Build history of the part. All positions in model axes, mm. A direction names the side the tool comes from. Round coordinates to 2 decimals unless told otherwise and drop trailing zeros. Write each loop counter-clockwise with the first axis right and the second up, starting at its lowest first coordinate (ties: lowest second). Pieces come first, ordered by that corner, then holes.
1) Flat gauge pins, fed straight in: pin 1 (1 mm diameter, centred on y = -5, z = 2, fed in from +X); pin 2 (10 mm diameter, centred on x = -15, y = 15, fed in from -Z); pin 3 (3 mm diameter, centred on x = 0, y = 0, fed in from -Z). Where does each tip first touch, or does it go through?
2) Pull direction X, two halves, no side cores. Call faces 1 (the cylindrical face through (9.977, 15.656, 1.282)), 2 (the cylindrical face through (14.54, -18.62, 1.28)), 3 (the cylindrical face through (-23.598, 1.206, 1.282)): +X half, -X half, draft (parallel to the pull), parting line (faces both ways), or undercut.
3) Saw through at A-A (x = 0). Write the cut outline in (y, z), plus the area to 3 significant figures.
4) Which spindle directions (+Z, -Z, +X, -X, +Y, -Y) get a long thin tool onto all of the face, cutting with end or side? Do faces 4 (the cylindrical face through (-10.9, -20.965, 1.282)), 5 (the cylindrical face through (8.71, 22.02, 1.28)). Say none if no direction does.
5) Saw through at C-C (y = 1.5). Write the cut outline in (x, z).
6) Saw through at B-B (y = 17). Write the cut outline in (x, z).
7) Saw through at D-D (x = 11). Write the cut outline in (y, z).
8) Wall check: probe 1 along X at (y, z) = (-2, 2.35); probe 2 along X at (y, z) = (-22, 1); probe 3 along X at (y, z) = (-1.5, 0.95). Give the ranges that are in metal, low to high.
from build123d import *

# Parameters (mm, degrees)
SK_DISCO_R           = 25.436113967
SK_DISCO_R_2         = 2.6
DISCO_DEPTH          = 2.6
HUECO_DIENTE_DEPTH   = 37.065936664
MATRIZ_DIENTES_COUNT = 11


with BuildPart() as part:
    # Sk_Disco → Disco (new body)
    with BuildSketch(Plane.XY):
        Circle(SK_DISCO_R)
        Circle(SK_DISCO_R_2, mode=Mode.SUBTRACT)
    extrude(amount=DISCO_DEPTH)

    # Sk_Hueco → Hueco_diente (cut, through all)
    with BuildSketch(Plane.XY):
        with BuildLine():
            ThreePointArc((-3.81398457, 21.41921922), (0, 18.564106134), (3.81398457, 21.41921922))
            ThreePointArc((3.81398457, 21.41921922), (5.23928173, 24.240764826), (7.576378688, 26.369278253))
            ThreePointArc((7.576378688, 26.369278253), (0, 27.436113967), (-7.576378688, 26.369278253))
            ThreePointArc((-7.576378688, 26.369278253), (-5.23928173, 24.240764826), (-3.81398457, 21.41921922))
        make_face()
    hueco_diente = extrude(amount=HUECO_DIENTE_DEPTH, mode=Mode.SUBTRACT)

    # Matriz_dientes: Hueco_diente ×11 about axis
    matriz_dientes_axis = Axis((0, 0, 0), (0, 0, 1))
    for i in range(1, MATRIZ_DIENTES_COUNT):
        add(hueco_diente.rotate(matriz_dientes_axis, i * 360 / MATRIZ_DIENTES_COUNT), mode=Mode.SUBTRACT)


solid = part.part
Evaluation:
1. pin 1: stops at x = 19.06
1. pin 2: stops at z = 0
1. pin 3: passes through
2. face 1: undercut
2. face 2: +X half
2. face 3: -X half
3. outline: (-25.44, 0) - (-2.6, 0) - (-2.6, 2.6) - (-25.44, 2.6) - close; (2.6, 0) - (18.56, 0) - (18.56, 2.6) - (2.6, 2.6) - close
3. area: 101 mm2
4. face 4: +Z, -Z, -Y
4. face 5: +Z, -Z, +X
5. outline: (-24.28, 0) - (-2.12, 0) - (-2.12, 2.6) - (-24.28, 2.6) - close; (2.12, 0) - (24.28, 0) - (24.28, 2.6) - (2.12, 2.6) - close
6. outline: (-18.92, 0) - (-16.28, 0) - (-16.28, 2.6) - (-18.92, 2.6) - close; (-8.73, 0) - (8.73, 0) - (8.73, 2.6) - (-8.73, 2.6) - close; (16.28, 0) - (18.92, 0) - (18.92, 2.6) - (16.28, 2.6) - close
7. outline: (-21.06, 0) - (15.17, 0) - (15.17, 2.6) - (-21.06, 2.6) - close
8. probe 1: x = -18.52 to -1.66, 1.66 to 18.52
8. probe 2: x = -12.77 to -12.16, -2.37 to 2.37, 12.16 to 12.77
8. probe 3: x = -18.72 to -2.12, 2.12 to 18.72
